Autodesk Inventor part; units mm, degrees
ref_plane "Work Plane2" through (29.464, 0, 0) normal (-1, 0, 0) x (0, 0, 1)
ref_plane "YZ Plane" through (0, 0, 0) normal (1, 0, 0) x (0, 1, 0)
ref_plane "XZ Plane" through (0, 0, 0) normal (0, 1, 0) x (-1, 0, 0)
sketch "Sketch8" plane through (10.3632, 0, 0) normal (0, 0, 1) x (0, 1, 0)
  line L0 (3.683, -14.2748) -> (0, -14.2748)
  line L1 (0, -14.2748) -> (0, 10.3632)
  line L2 (0, -14.2748) -> (3.683, -14.2748)
  line L3 (3.683, 4.7752) -> (2.6124, 4.7752)
  line L4 (2.6124, 10.3632) -> (0, 10.3632)
  line L5 (2.6124, 10.3632) -> (3.683, 4.7752)
  line L6 (2.6124, 4.7752) -> (3.683, -0.0508)
  line L7 (2.6124, -0.0508) -> (3.683, -4.8768)
  line L8 (3.683, -0.0508) -> (2.6124, -0.0508)
  line L9 (3.683, -4.8768) -> (2.6124, -4.8768)
  line L10 (2.6124, -4.8768) -> (3.683, -9.7028)
  line L11 (3.683, -9.7028) -> (2.6687, -9.7028)
  line L12 (2.6687, -9.7028) -> (3.683, -14.2748)
  point P0 (0, 10.3632)
  dimension "d67" = 7.366
  dimension "d68" = 5.588
  dimension "d66" = 4.826
  dimension "d65" = 4.826
  dimension "d64" = 4.826
  dimension "d69" = 5.2248
  dimension "d87" = 24.638
revolve "Revolution5" add sketch "Sketch8" angle 360 about axis through (24.638, 0, 0) along (-1, 0, 0)
sketch "Sketch1" plane through (24.638, 0, 0) normal (1, 0, 0) x (0, 0, -1)
  line L0 (7.1437, 4.1244) -> (7.1438, -4.1244)
  line L1 (7.1438, -4.1244) -> (0, -8.2489)
  line L2 (0, -8.2489) -> (-7.1437, -4.1244)
  line L3 (-7.1437, -4.1244) -> (-7.1437, 4.1244)
  line L4 (-7.1437, 4.1244) -> (0, 8.2489)
  line L5 (0, 8.2489) -> (7.1437, 4.1244)
  circle A0 centre (0, 0) radius 3.683
  dimension "d51" = 14.2875
extrude "Extrusion1" add sketch "Sketch1" along normal blind 4.826 contours L0 L1 L2 L3 L4 L5 | A0
sketch "Sketch6" plane through (0, 0, 0) normal (0, 0, 1) x (1, 0, 0)
  line L0 (-8.7376, 0) -> (52.4256, 0)
  line L1 (29.464, -4.1244) -> (29.464, 4.1244)
  line L2 (29.464, 0) -> (29.464, 7.1437)
  line L3 (29.464, 7.1437) -> (43.688, 7.1437)
  line L4 (43.688, 7.1437) -> (43.688, 0)
  line L5 (29.464, 0) -> (43.688, 0)
  line L6 (0, -2.6124) -> (0, 2.6124)
  dimension "d73" = 14.2875
  dimension "d74" = 43.688
revolve "Revolution3" add sketch "Sketch6" angle 360 about axis through (-10, 0, 0) along (1, 0, 0)
chamfer "Chamfer1" distance 0.475 angle 45 1 edges at (43.688, -7.1437, 0)
sketch "Sketch7" plane through (0, 0, 0) normal (0, 1, 0) x (-1, 0, 0)
  line L0 (-24.638, 7.1437) -> (-24.638, 10.7156)
  line L1 (-24.638, 10.7156) -> (-26.3036, 10.7156)
  line L2 (-26.3036, 10.7156) -> (-24.638, 7.1437)
  line L3 (-29.464, 7.1437) -> (-29.464, 10.7156)
  line L4 (-29.464, 10.7156) -> (-27.7984, 10.7156)
  line L5 (-27.7984, 10.7156) -> (-29.464, 7.1437)
  line L6 (-23.6728, 0) -> (-30.4292, 0)
  dimension "d75" = 3.5719
  dimension "d76" = 25
revolve "Revolution4" cut sketch "Sketch7" angle 360 about axis through (-10, 0, 0) along (1, 0, 0)
hole "Hole1" at (43.688, 0, 0) direction (-1, 0, 0) diameter 5.6998 depth 13.1064 countersink diameter 6.4122 countersink angle 82
hole "Hole2" at (30.5816, 0, 0) direction (-1, 0, 0) diameter 4.7498 end through all countersink diameter 5.6998 countersink angle 82
sketch "Sketch9" plane through (0, 0, 0) normal (0, 0, 1) x (1, 0, 0)
  line L0 (30.5562, 6.4654) -> (30.5562, -9.2124)
  line L1 (29.464, 0) -> (29.464, -6.1867)
  dimension "d86" = 1.0922
split_face "Split1"
thread "Rosca1"
ref_plane "Work Plane2" through (29.464, 0, 0) normal (-1, 0, 0) x (0, 0, 1)
equation "\"d67\" = OD"
equation "\"d68\" = L1"
equation "\"d66\" = L2"
equation "\"d65\" = L2"
equation "\"d64\" = L2"
equation "\"d69\" = 1.1 * D1"
equation "\"d87\" = M"
equation "\"d51\" = C_HEX"
equation "\"d1\" = C_HEX_L"
equation "\"d73\" = C_HEX"
equation "\"d74\" = L"
equation "\"d37\" = 0.1 * D1"
equation "\"d75\" = 0.25 * C_HEX"
equation "\"d54\" = 1.2 * D1"
equation "\"d56\" = 1.35 * D1"
equation "\"d59\" = 0.3 * L"
equation "\"d79\" = D1"
equation "\"d81\" = 1.2 * D1"
equation "\"d86\" = 0.025 * L"
equation "\"C_HEX\" = 14.2875"
equation "\"L\" = 43.688"
equation "\"M\" = 24.638"
equation "\"OD\" = 7.366"
equation "\"D1\" = 4.7498"
equation "\"d6\" = 0.2 * M"
equation "\"d7\" = 0.2 * M"
equation "\"d8\" = 0.2 * M"
equation "\"d9\" = 0.2 * M"
equation "\"L1\" = 5.588"
equation "\"L2\" = 4.826"
equation "\"C_HEX_L\" = 4.826"
equation "\"d88\" = -C_HEX_L"
equation "\"Parker_No\" = 1.2345"
properties part number "Terminación de manguera para tubería macho 125HBL de Parker 125HBL-4-4" material "Latón, amarillo claro"
For this review, take the finished solid that the model builds, in its own axes (mm). A direction names the side the tool comes from. Give positions to 0.01 mm unless a question says otherwise; leave off trailing zeros. Write each loop counter-clockwise with the first axis right and the second up, starting at its lowest first coordinate (ties: lowest second). Pieces come first, ordered by that corner, then holes. Notation, with made-up numbers: M 18,11 L 38,11 A14 ccw 38,35 Z; hole C 32,47 d3. An arc over 180 degrees is marked long. One line per item, written item: value.
1) For P1, Ø8, axis at x = 35, z = -5.5, coming from the +Y side; P2, Ø2, axis at y = -0.5, z = 1.5, coming from the +X side; P3, Ø5.5, axis at y = 0, z = 0, coming from the -X side; P4, Ø2, axis at y = -1.5, z = -1, coming from the +X side, all flat-tipped, find the tip position at first contact; note any pin that passes through.
Results are:
P1: stops at y = 6.98
P2: stops at x = 30.27
P3: stops at x = 0
P4: stops at x = 30.53
2) For line 1 (Z direction, x = 39.5, y = 0); line 2 (Z direction, x = 24, y = 0), list the stretches that pass through material, from the lowest coordinate up. Write a range as from..to.
Results are:
line 1: z = -7.14..-2.85, 2.85..7.14
line 2: z = -3.54..-2.37, 2.37..3.54
3) Take a section at A-A, the plane x = 18. Write out the cut boundary in (y, z).
Results are:
outline: C 0,0 d6.45; hole C 0,0 d4.75
4) For faces 1 (the cylindrical face through (36.435, 6.814, 2.146)), 2 (the conical face through (21.876, -0.4, 3.044)), 3 (the flat face through (27.02, -6.16, -3.62)), 4 (the flat face through (24.638, -3, -3)), list the 3-axis set-ups (+Z, -Z, +X, -X, +Y, -Y) from which the entire face can be reached by the end or side of a thin tool; tool diameter is ignored.
Results are:
face 1: +X
face 2: none
face 3: -Z, +X, -X, -Y
face 4: -X
5) The part is to be moulded in two halves that separate along Y. For faces 5 (the cylindrical face through (36.841, -0.856, -2.718)), 6 (the flat face through (27.017, -6.216, 3.522)), 7 (the flat face through (10.414, 1, -3)), say which applies: +Y half, -Y half, draft (parallel to the pull), parting line (faces both ways), or undercut.
Results are:
face 5: undercut
face 6: -Y half
face 7: draft
